Design review of the part built by this model. Coordinates are the model's own, in mm. Face numbers are marked on the shaded views. A direction names the side the tool comes from. Coordinates: 2 decimals unless noted, no trailing zeros. Loops run counter-clockwise (first coordinate to the right, second up) from the corner with the lowest first, then second, coordinate; pieces in that order, holes last.
Q1. Machinability: for the marked faces 4 and 5, which of the approach directions +Z, -Z, +X, -X, +Y, -Y give a long, thin tool a straight path to every point of the face, cutting with its end or side? Answer none if there is none.
Q2. Add section D-D on x = -51. Give the boundary of the cut face in (y, z), and give its area (3 significant figures).
Q3. Add section B-B on y = 36.5. Give the boundary of the cut face in (x, z).
Q4. Draft analysis for pull direction Y (two halves, no side actions). For the marked faces 1, 2 and 3, state which applies: released by +Y, released by -Y, zero draft, split by the parting line, or undercut.
Q5. Add section A-A on x = -28. Give the boundary of the cut face in (y, z).
Q6. Wall thickness on probe 1 along X at (y, z) = (-18, 4); probe 2 along X at (y, z) = (-14.5, 5.5); probe 3 along Y at (x, z) = (0, 1.5): over which ranges is each line inside the solid? List them lowest first.
Q7. Add section C-C on z = 4.25. Give the boundary of the cut face in (x, y).
Q8. For P1, Ø4, axis at x = -42.5, z = 3.5, coming from the +Y side; P2, Ø4, axis at x = -21, z = 2.5, coming from the +Y side; P3, Ø1, axis at y = 15.5, z = 1.5, coming from the +X side, all flat-tipped, find the tip position at first contact; note any pin that passes through.
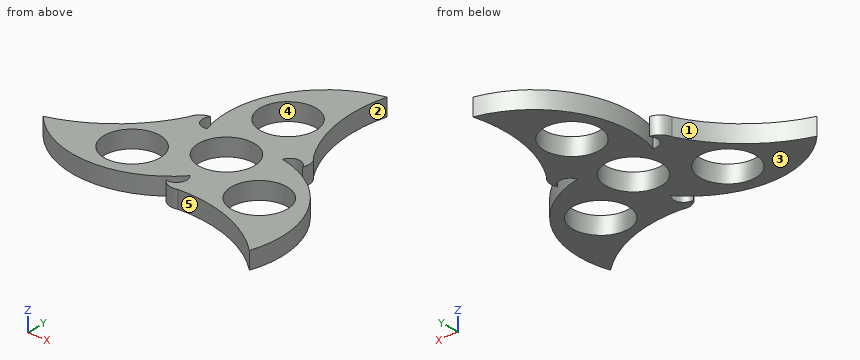
```python
from build123d import *

# Parameters (mm, degrees)
F0_R     = 11.2
F1_DEPTH = 7


with BuildPart() as f1:
    # F0 (on Top) → F1 (new body)
    with BuildSketch(Plane.XY):
        with BuildLine():
            ThreePointArc((-24.555476, 10.805503), (-38.89385, -6.957617), (-59.095755, -17.587779))
            ThreePointArc((-59.095755, -17.587779), (-29.547878, -30.85808), (0, -17.587779))
            ThreePointArc((0, -17.587779), (0.616641, -22.365553), (-3.718256, -24.466991))
            ThreePointArc((-3.718256, -24.466991), (-0.778036, -26.710105), (2.919898, -26.668418))
            ThreePointArc((2.919898, -26.668418), (25.472398, -30.204253), (44.779341, -42.384536))
            ThreePointArc((44.779341, -42.384536), (41.49782, -10.160173), (15.231463, 8.79389))
            ThreePointArc((15.231463, 8.79389), (19.060817, 11.716804), (23.048163, 9.013391))
            ThreePointArc((23.048163, 9.013391), (23.520647, 12.681254), (21.635578, 15.862915))
            ThreePointArc((21.635578, 15.862915), (13.421452, 37.16187), (14.316414, 59.972315))
            ThreePointArc((14.316414, 59.972315), (-11.949942, 41.018252), (-15.231463, 8.79389))
            ThreePointArc((-15.231463, 8.79389), (-19.677458, 10.64875), (-19.329907, 15.453599))
            ThreePointArc((-19.329907, 15.453599), (-22.742611, 14.028851), (-24.555476, 10.805503))
        make_face()
        with Locations((-25.58171, -14.769607)):
            Circle(F0_R, mode=Mode.SUBTRACT)
        Circle(F0_R, mode=Mode.SUBTRACT)
        with Locations((25.58171, -14.769607)):
            Circle(F0_R, mode=Mode.SUBTRACT)
        with Locations((0, 29.539214)):
            Circle(F0_R, mode=Mode.SUBTRACT)
    extrude(amount=F1_DEPTH)


solid = f1.part
```
Entries:
1. face 4: +Z, -Z
1. face 5: +Z, -Z, -Y
2. outline: (-24.53, 0) - (-14.56, 0) - (-14.56, 7) - (-24.53, 7) - close
2. area: 69.8 mm2
3. outline: (-14.19, 0) - (-8.77, 0) - (-8.77, 7) - (-14.19, 7) - close; (8.77, 0) - (13.54, 0) - (13.54, 7) - (8.77, 7) - close
4. face 1: released by +Y
4. face 2: undercut
4. face 3: zero draft
5. outline: (-30.83, 0) - (-25.71, 0) - (-25.71, 7) - (-30.83, 7) - close; (-3.83, 0) - (5, 0) - (5, 7) - (-3.83, 7) - close
6. probe 1: x = -58.72 to -36.31, -14.86 to -0.37, 0.34 to 14.86, 36.31 to 44.95
6. probe 2: x = -50.86 to -36.78, -14.38 to 14.38, 36.78 to 43.66
6. probe 3: y = -26.91 to -23.22, -17.59 to -11.2, 11.2 to 18.34, 40.74 to 53.9
7. outline: (-59.1, -17.59) arc R39.53 ccw to (0, -17.59) arc R4.12 cw to (-3.72, -24.47) arc R5.68 ccw to (2.92, -26.67) arc R56.44 cw to (44.78, -42.38) arc R39.53 ccw to (15.23, 8.79) arc R4.12 cw to (23.05, 9.01) arc R5.68 ccw to (21.64, 15.86) arc R56.44 cw to (14.32, 59.97) arc R39.53 ccw to (-15.23, 8.79) arc R4.12 cw to (-19.33, 15.45) arc R5.68 ccw to (-24.56, 10.81) arc R56.44 cw to start; hole circle Ø22.4 at (-25.58, -14.77); hole circle Ø22.4 at (0, 0); hole circle Ø22.4 at (0, 29.54); hole circle Ø22.4 at (25.58, -14.77)
8. P1: stops at y = -8.23
8. P2: stops at y = 15.45
8. P3: stops at x = 22.46
